The listing builds one solid part. Answer for the finished solid, in the listing's coordinates (mm). Face numbers are marked on the shaded views. A direction names the side the tool comes from. Give positions to 0.01 mm unless a question says otherwise; leave off trailing zeros. Write each loop counter-clockwise with the first axis right and the second up, starting at its lowest first coordinate (ties: lowest second). Pieces come first, ordered by that corner, then holes. Notation, with made-up numbers: (35, 53.5) - (82, 53.5) arc R17 ccw to (82, 58.5) - close; hole circle Ø9 at (41.5, -10). An arc over 180 degrees is marked (long way). One line per question, with ' | ' between items. Start each with the question number.
1. A cutting plane is placed at A-A (x = -23). Determine the outline of the cut face in (y, z), then the cut area to 3 significant figures.
2. A cutting plane is placed at C-C (y = -12). Determine the outline of the cut face in (x, z).
3. A cutting plane is placed at B-B (z = 1). Determine the outline of the cut face in (x, y).
4. Given P1, Ø7.5, axis at x = -26, y = -39.5, coming from the +Z side; P2, Ø6, axis at x = 15, z = -0.5, coming from the +Y side; P3, Ø4, axis at x = 7, y = -12.5, coming from the +Z side; P4, Ø12, axis at x = -18.5, z = 2.5, coming from the -Y side, each flat-ended and moving along its own axis, determine where each tip first touches the part or whether it passes through.
5. For the marked faces 1, 2, 3, 4 and 5, determine the directions among +Z, -Z, +X, -X, +Y, -Y from which every point of the face is accessible in a straight line to the end or side of a thin tool.
6. A cutting plane is placed at D-D (z = 13.5). Determine the outline of the cut face in (x, y).
7. Find the intervals of material crossed by L1, parallel to Y at x = 9.5, z = -9; L2, parallel to X at y = -40.5, z = -20; L3, parallel to X at y = -47.5, z = -10.5, in increasing order. Write a range as from..to.
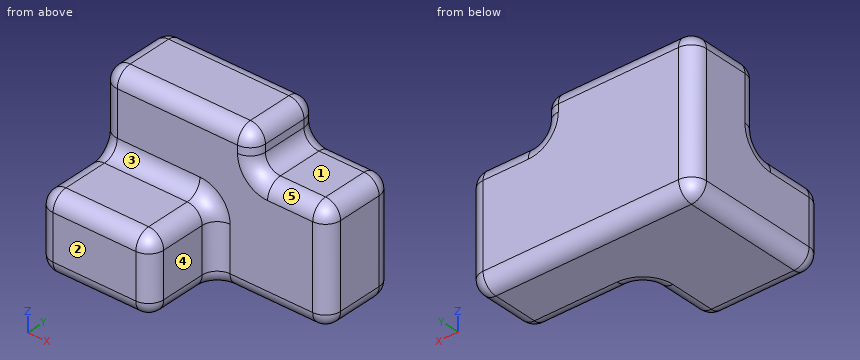
```python
from build123d import *

# Parameters (mm, degrees)
F1_DEPTH = 25.4
F2_W     = 38.1
F2_H     = 25.4
F3_DEPTH = 25.4
F4_R     = 5.08


with BuildPart() as f1:
    # F0 (on Front) → F1 (new body)
    with BuildSketch(Plane.XZ):
        Polygon((6.5013106585, 19.9951574836), (-44.2986893415, 19.9951574836), (-44.2986893415, -30.8048425164), (31.9013106585, -30.8048425164), (31.9013106585, 7.2951574836), (6.5013106585, 7.2951574836), align=None)
    extrude(amount=F1_DEPTH)

    # F2 (on face) → F3 (join)
    with BuildSketch(Plane.XZ.offset(25.4)):
        with Locations((-25.2486893415, -18.1048425164)):
            Rectangle(F2_W, F2_H)
    extrude(amount=F3_DEPTH)

    # F4
    f4_edges = [f1.edges().sort_by_distance(p)[0] for p in [
        (6.501311, -12.7, 19.995157),
        (-44.298689, -12.7, 19.995157),
        (-18.898689, 0, 19.995157),
        (-18.898689, -25.4, 19.995157),
        (31.901311, -12.7, 7.295157),
        (6.501311, -12.7, 7.295157),
        (19.201311, 0, 7.295157),
        (19.201311, -25.4, 7.295157),
        (-6.198689, -50.8, -18.104843),
        (-25.248689, -50.8, -5.404843),
        (-44.298689, -50.8, -18.104843),
        (-25.248689, -50.8, -30.804843),
        (-6.198689, -38.1, -5.404843),
        (-44.298689, -38.1, -5.404843),
        (-25.248689, -25.4, -5.404843),
        (-6.198689, -38.1, -30.804843),
        (-6.198689, -25.4, -18.104843),
        (31.901311, -12.7, -30.804843),
        (31.901311, 0, -11.754843),
        (31.901311, -25.4, -11.754843),
        (12.851311, -25.4, -30.804843),
        (-44.298689, -25.4, 7.295157),
        (6.501311, -25.4, 13.645157),
        (6.501311, 0, 13.645157),
        (-44.298689, 0, -5.404843),
        (-6.198689, 0, -30.804843),
        (-44.298689, -25.4, -30.804843),
    ]]
    fillet(f4_edges, radius=F4_R)


solid = f1.part
```
Determined:
1) outline: (-50.8, -25.72) arc R5.08 ccw to (-45.72, -30.8) - (-5.08, -30.8) arc R5.08 ccw to (0, -25.72) - (0, 14.92) arc R5.08 ccw to (-5.08, 20) - (-20.32, 20) arc R5.08 ccw to (-25.4, 14.92) - (-25.4, -0.32) arc R5.08 cw to (-30.48, -5.4) - (-45.72, -5.4) arc R5.08 ccw to (-50.8, -10.48) - close | area: 1,910 mm2
2) outline: (-44.3, -25.72) arc R5.08 ccw to (-39.22, -30.8) - (26.82, -30.8) arc R5.08 ccw to (31.9, -25.72) - (31.9, 2.22) arc R5.08 ccw to (26.82, 7.3) - (11.58, 7.3) arc R5.08 cw to (6.5, 12.38) - (6.5, 14.92) arc R5.08 ccw to (1.42, 20) - (-39.22, 20) arc R5.08 ccw to (-44.3, 14.92) - close
3) outline: (-44.3, -20.32) arc R5.08 ccw to (-39.22, -25.4) - (26.82, -25.4) arc R5.08 ccw to (31.9, -20.32) - (31.9, -5.08) arc R5.08 ccw to (26.82, 0) - (-39.22, 0) arc R5.08 ccw to (-44.3, -5.08) - close
4) P1: z = -5.4 | P2: y = 0 | P3: z = 18.52 | P4: y = -26.51
5) face 1: +Z, +X, +Y, -Y | face 2: +Z, -Z, +X, -X, -Y | face 3: +Z, +X, -X, -Y | face 4: +Z, -Z, +X, -Y | face 5: +Z, +X, -Y
6) outline: (-44.3, -20.32) arc R5.08 ccw to (-39.22, -25.4) - (1.42, -25.4) arc R5.08 ccw to (6.5, -20.32) - (6.5, -5.08) arc R5.08 ccw to (1.42, 0) - (-39.22, 0) arc R5.08 ccw to (-44.3, -5.08) - close
7) L1: -25.4..0 | L2: -44.3..-6.2 | L3: -43.98..-6.52
